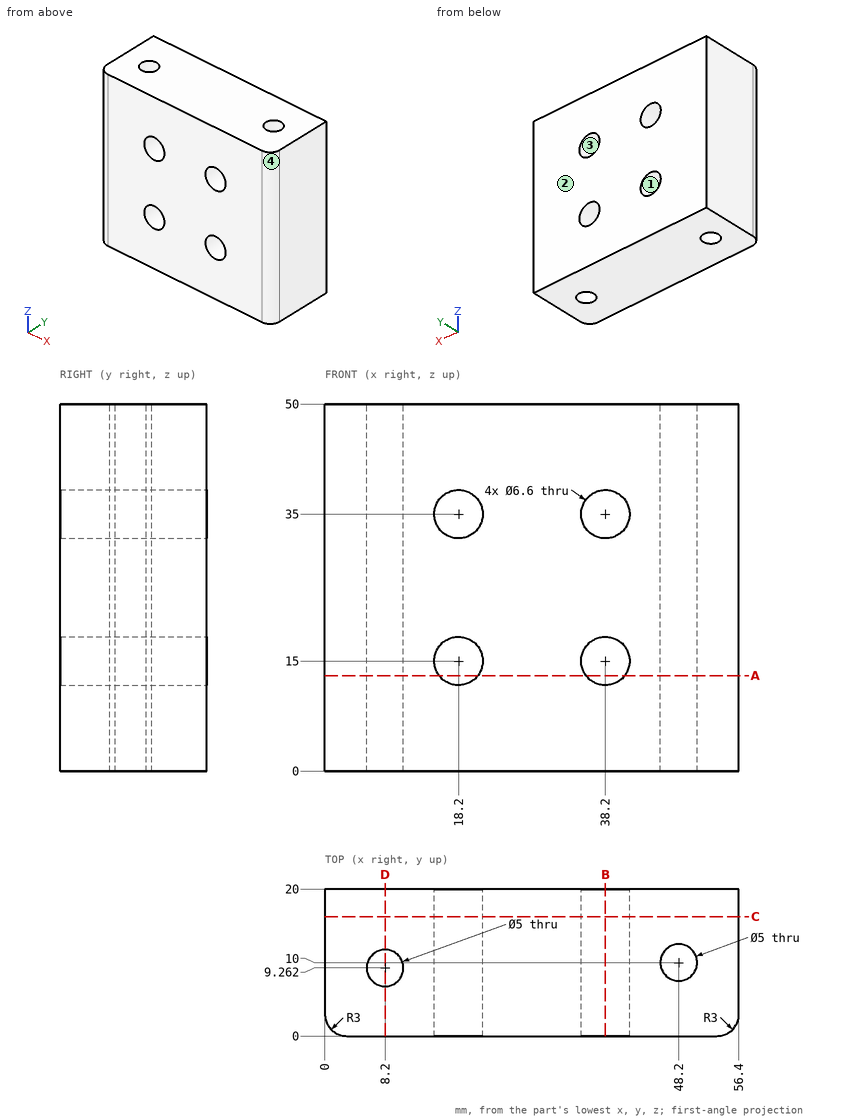
For this review, use the dimensioned drawing (mm, ordinates from the lowest corner) and the shaded views. Give positions to 0.01 mm unless a question says otherwise; leave off trailing zeros. Order: outer loops, then holes, each group sorted by start corner. A loop starts at its lowest first (then second) coordinate and runs counter-clockwise, first axis right, second up. Notation, with made-up numbers: (36, 54) -> (68, 54) arc R15 cw to (68, 74) -> close; hole circle Ø6 at (30.5, -30). An arc over 180 degrees is marked (long way). Write item = value, one per line. Start each with the question number.
(1) Take a section at A-A (z = 13). Write out the cut boundary in (x, y) (1 decimal).
(2) For L1, parallel to Z at x = 18.2, y = 10; L2, parallel to Y at x = 8, z = 32 (1 decimal); L3, parallel to Z at x = 37, y = 5.75 (1 decimal), list the stretches that pass through material, from the lowest coordinate up. Write a range as from..to.
(3) Take a section at B-B (x = 38.2). Write out the cut boundary in (y, z).
(4) Draft analysis for pull direction X (two halves, no side actions). For the marked faces 1, 2, 3 and 4, state which applies: +X half, -X half, draft (parallel to the pull), parting line (faces both ways), or undercut.
(5) For pin 1 Ø3 at (x, y) = (8.2, 9.26) entering from +Z; pin 2 Ø6 at (x, y) = (14, 13) entering from -Z, all flat-tipped, find the tip position at first contact; note any pin that passes through.
(6) Take a section at D-D (x = 8.2). Write out the cut boundary in (y, z), plus the area to 3 significant figures.
(7) Take a section at C-C (y = 16.25). Write out the cut boundary in (x, z).
Returned:
q1.outline = (0, 3) arc R3 ccw to (3, 0) -> (15.6, 0) -> (15.6, 20) -> (0, 20) -> close; (20.8, 0) -> (35.6, 0) -> (35.6, 20) -> (20.8, 20) -> close; (40.8, 0) -> (53.4, 0) arc R3 ccw to (56.4, 3) -> (56.4, 20) -> (40.8, 20) -> close; hole circle Ø5 at (8.2, 9.3); hole circle Ø5 at (48.2, 10)
q2.L1 = 0..11.7, 18.3..31.7, 38.3..50
q2.L2 = 0..6.8, 11.8..20
q2.L3 = 0..11.9, 18.1..31.9, 38.1..50
q3.outline = (0, 0) -> (20, 0) -> (20, 11.7) -> (0, 11.7) -> close; (0, 18.3) -> (20, 18.3) -> (20, 31.7) -> (0, 31.7) -> close; (0, 38.3) -> (20, 38.3) -> (20, 50) -> (0, 50) -> close
q4.face_1 = undercut
q4.face_2 = draft
q4.face_3 = undercut
q4.face_4 = +X half
q5.pin_1 = through
q5.pin_2 = 0
q6.outline = (0, 0) -> (6.76, 0) -> (6.76, 50) -> (0, 50) -> close; (11.76, 0) -> (20, 0) -> (20, 50) -> (11.76, 50) -> close
q6.area = 750 mm²
q7.outline = (0, 0) -> (56.4, 0) -> (56.4, 50) -> (0, 50) -> close; hole circle Ø6.6 at (18.2, 15); hole circle Ø6.6 at (18.2, 35); hole circle Ø6.6 at (38.2, 15); hole circle Ø6.6 at (38.2, 35)
